from build123d import *


with BuildPart() as f1:
    # F0 (on Front) → F1 (revolve)
    with BuildSketch(Plane.XZ):
        with BuildLine():
            Line((12.5984, 13.3858), (11.5062, 13.3858))
            Line((11.5062, 13.3858), (11.5062, 14.9606))
            Line((11.5062, 14.9606), (12.5984, 14.9606))
            Line((12.5984, 14.9606), (12.5984, 22.44372))
            ThreePointArc((12.5984, 22.44372), (11.680449, 24.659849), (9.46432, 25.5778))
            Line((9.46432, 25.5778), (0, 25.5778))
            Line((0, 25.5778), (0, -28.1051))
            Line((0, -28.1051), (12.7, -28.1051))
            Line((12.7, -28.1051), (12.7, -15.1003))
            Line((12.7, -15.1003), (11.02614, -15.1003))
            Line((11.02614, -15.1003), (11.02614, -13.5255))
            Line((11.02614, -13.5255), (12.5984, -13.5255))
            Line((12.5984, -13.5255), (12.5984, 13.3858))
        make_face()
    revolve(axis=Axis((0, 0, -1.26365), (0, 0, -1)))


solid = f1.part
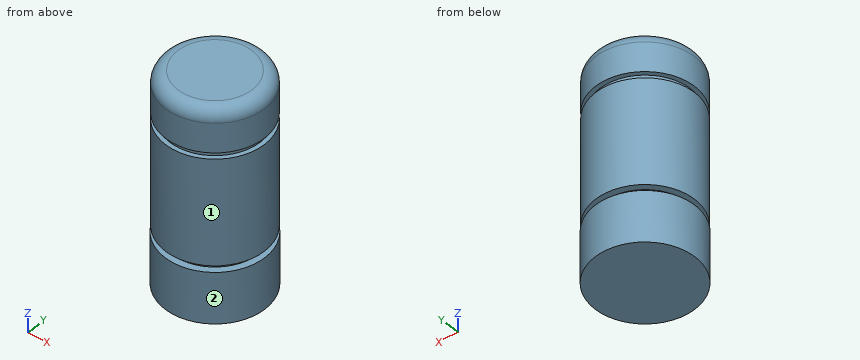
Could you check a few things on this model? Use its own coordinates, in mm. Face numbers are marked on the shaded views. A direction names the side the tool comes from. Round coordinates to 2 decimals unless told otherwise and drop trailing zeros. Write each loop counter-clockwise with the first axis right and the second up, starting at its lowest first coordinate (ties: lowest second). Pieces come first, ordered by that corner, then holes. Notation, with made-up numbers: (16, 23) -> (38, 23) arc R13 cw to (38, 43) -> close; hole circle Ø11 at (81, 71.25). An arc over 180 degrees is marked (long way). Use a Markdown table: item, result.
1. Which directions (+Z, -Z, +X, -X, +Y, -Y) give clear straight access to the entire face, cutting with the end or side of a thin tool? Please do the marked faces 1 and 2.
Answer key:
| item | result |
|---|---|
| face 1 | +Z |
| face 2 | +Z, -Z |
2. For pin 1 Ø8 at (y, z) = (-1, -2) entering from +X; pin 2 Ø12 at (y, z) = (-9.5, -1) entering from +X; pin 3 Ø4 at (x, z) = (-3.5, 13.5) entering from -Y, each with a flat end and sliding along its axis, tell me the tip position at first contact or that it passes through.
Answer key:
| item | result |
|---|---|
| pin 1 | stops at x = 12.6 |
| pin 2 | stops at x = 12.1 |
| pin 3 | stops at y = -12.51 |
3. If we section it at A-A (x = 0): List the corners of the cut face in (y, z) for me.
Answer key:
| item | result |
|---|---|
| outline | (-12.7, -28.11) -> (12.7, -28.11) -> (12.7, -15.1) -> (11.03, -15.1) -> (11.03, -13.53) -> (12.6, -13.53) -> (12.6, 13.39) -> (11.51, 13.39) -> (11.51, 14.96) -> (12.6, 14.96) -> (12.6, 22.44) arc R3.13 ccw to (9.46, 25.58) -> (-9.46, 25.58) arc R3.13 ccw to (-12.6, 22.44) -> (-12.6, 14.96) -> (-11.51, 14.96) -> (-11.51, 13.39) -> (-12.6, 13.39) -> (-12.6, -13.53) -> (-11.03, -13.53) -> (-11.03, -15.1) -> (-12.7, -15.1) -> close |
4. If we section it at C-C (z = 11): List the corners of the cut face in (x, y) for me, then the cut area to 3 significant figures.
Answer key:
| item | result |
|---|---|
| outline | circle Ø25.2 at (0, 0) |
| area | 499 mm^2 |
5. Please list where these lines run through material, in increasing order: probe 1 along Z at (x, y) = (-10.75, 4.5); probe 2 along Z at (x, y) = (7.5, -6); probe 3 along Z at (x, y) = (-11.25, -4).
Answer key:
| item | result |
|---|---|
| probe 1 | z = -28.11 to -15.1, -13.53 to 13.39, 14.96 to 24.69 |
| probe 2 | z = -28.11 to 25.57 |
| probe 3 | z = -28.11 to -15.1, -13.53 to 13.39, 14.96 to 24.37 |
